from build123d import *

# Parameters (mm, degrees)
ESQUISSE1_W             = 90
ESQUISSE1_H             = 40
ESQUISSE1_R             = 5.05
ESQUISSE1_R_2           = 1.75
BOSS_EXTRU_1_DEPTH      = 10
ESQUISSE3_W             = 80
ESQUISSE3_H             = 40
ENL_V_MAT_EXTRU_3_DEPTH = 5
ESQUISSE4_R             = 1.75
BOSS_EXTRU_2_DEPTH      = 10
ESQUISSE2_R             = 1.75
ENL_V_MAT_EXTRU_1_DEPTH = 5
ENL_V_START             = -85
ESQUISSE2_2_R           = 1.75
ENL_V_MAT_EXTRU_2_DEPTH = 5
BOSS_EXTRU_3_START      = 10
ESQUISSE5_W             = 10
ESQUISSE5_H             = 50
ESQUISSE5_R             = 1.75
BOSS_EXTRU_3_DEPTH      = 10
BOSS_EXTRU_4_START      = -100
ESQUISSE5_2_W           = 10
ESQUISSE5_2_H           = 50
ESQUISSE5_2_R           = 1.75
BOSS_EXTRU_4_DEPTH      = 10
ESQUISSE6_R             = 1.75
ENL_V_MAT_EXTRU_4_DEPTH = 10
ESQUISSE7_R             = 5.05
ESQUISSE7_R_2           = 4.05
BOSS_EXTRU_5_DEPTH      = 2
ESQUISSE8_R             = 8
ESQUISSE8_R_2           = 5.05
BOSS_EXTRU_6_DEPTH      = 1.8


with BuildPart() as part:
    # Esquisse1 → Boss.-Extru.1 (new body)
    with BuildSketch(Plane.XY):
        with Locations((45, 20)):
            Rectangle(ESQUISSE1_W, ESQUISSE1_H)
        with Locations((45, 19)):
            Circle(ESQUISSE1_R, mode=Mode.SUBTRACT)
        with Locations((15, 35)):
            Circle(ESQUISSE1_R_2, mode=Mode.SUBTRACT)
        with Locations((25, 35)):
            Circle(ESQUISSE1_R_2, mode=Mode.SUBTRACT)
        with Locations((35, 35)):
            Circle(ESQUISSE1_R_2, mode=Mode.SUBTRACT)
        with Locations((55, 35)):
            Circle(ESQUISSE1_R_2, mode=Mode.SUBTRACT)
        with Locations((65, 35)):
            Circle(ESQUISSE1_R_2, mode=Mode.SUBTRACT)
        with Locations((75, 35)):
            Circle(ESQUISSE1_R_2, mode=Mode.SUBTRACT)
        with Locations((15, 25)):
            Circle(ESQUISSE1_R_2, mode=Mode.SUBTRACT)
        with Locations((25, 25)):
            Circle(ESQUISSE1_R_2, mode=Mode.SUBTRACT)
        with Locations((65, 25)):
            Circle(ESQUISSE1_R_2, mode=Mode.SUBTRACT)
        with Locations((75, 25)):
            Circle(ESQUISSE1_R_2, mode=Mode.SUBTRACT)
        with Locations((15, 15)):
            Circle(ESQUISSE1_R_2, mode=Mode.SUBTRACT)
        with Locations((25, 15)):
            Circle(ESQUISSE1_R_2, mode=Mode.SUBTRACT)
        with Locations((65, 15)):
            Circle(ESQUISSE1_R_2, mode=Mode.SUBTRACT)
        with Locations((75, 15)):
            Circle(ESQUISSE1_R_2, mode=Mode.SUBTRACT)
        with Locations((15, 5)):
            Circle(ESQUISSE1_R_2, mode=Mode.SUBTRACT)
        with Locations((25, 5)):
            Circle(ESQUISSE1_R_2, mode=Mode.SUBTRACT)
        with Locations((35, 5)):
            Circle(ESQUISSE1_R_2, mode=Mode.SUBTRACT)
        with Locations((45, 5)):
            Circle(ESQUISSE1_R_2, mode=Mode.SUBTRACT)
        with Locations((55, 5)):
            Circle(ESQUISSE1_R_2, mode=Mode.SUBTRACT)
        with Locations((65, 5)):
            Circle(ESQUISSE1_R_2, mode=Mode.SUBTRACT)
        with Locations((75, 5)):
            Circle(ESQUISSE1_R_2, mode=Mode.SUBTRACT)
    extrude(amount=BOSS_EXTRU_1_DEPTH)

    # Esquisse3 → Enlèv. mat.-Extru.3 (cut)
    with BuildSketch(Plane.XY.offset(10)):
        with Locations((45, 20)):
            Rectangle(ESQUISSE3_W, ESQUISSE3_H)
    extrude(amount=-ENL_V_MAT_EXTRU_3_DEPTH, mode=Mode.SUBTRACT)

    # Esquisse4 → Boss.-Extru.2 (add)
    with BuildSketch(Plane.XZ):
        Polygon((0, 0), (0, 10), (10, 10), (10, 5), (80, 5), (80, 10), (90, 10), (90, 0), align=None)
        with Locations((5, 5)):
            Circle(ESQUISSE4_R, mode=Mode.SUBTRACT)
        with Locations(Location((85, 5, 0), (0, 0, 180))):
            Circle(ESQUISSE4_R, mode=Mode.SUBTRACT)
    extrude(amount=BOSS_EXTRU_2_DEPTH)

    # Esquisse2 → Enlèv. mat.-Extru.1 (cut)
    with BuildSketch(Plane(origin=(90, 0, 0), x_dir=(0, 0, -1), z_dir=(1, 0, 0))):
        with Locations(Location((-5, 35, 0), (0, 0, 90))):
            Circle(ESQUISSE2_R)
        with Locations(Location((-5, 25, 0), (0, 0, 90))):
            Circle(ESQUISSE2_R)
        with Locations(Location((-5, 15, 0), (0, 0, 90))):
            Circle(ESQUISSE2_R)
        with Locations(Location((-5, 5, 0), (0, 0, 90))):
            Circle(ESQUISSE2_R)
        with Locations(Location((-5, -5, 0), (0, 0, 90))):
            Circle(ESQUISSE2_R)
    extrude(amount=-ENL_V_MAT_EXTRU_1_DEPTH, mode=Mode.SUBTRACT)

    # Esquisse2<2> → Enlèv. mat.-Extru.2 (cut)
    with BuildSketch(Plane(origin=(90, 0, 0), x_dir=(0, 0, -1), z_dir=(1, 0, 0)).offset(ENL_V_START)):
        with Locations(Location((-5, 35, 0), (0, 0, 90))):
            Circle(ESQUISSE2_2_R)
        with Locations(Location((-5, 25, 0), (0, 0, 90))):
            Circle(ESQUISSE2_2_R)
        with Locations(Location((-5, 15, 0), (0, 0, 90))):
            Circle(ESQUISSE2_2_R)
        with Locations(Location((-5, 5, 0), (0, 0, 90))):
            Circle(ESQUISSE2_2_R)
        with Locations(Location((-5, -5, 0), (0, 0, 90))):
            Circle(ESQUISSE2_2_R)
    extrude(amount=-ENL_V_MAT_EXTRU_2_DEPTH, mode=Mode.SUBTRACT)

    # Esquisse5 → Boss.-Extru.3 (add)
    with BuildSketch(Plane(origin=(90, 0, 0), x_dir=(0, 0, -1), z_dir=(1, 0, 0)).offset(BOSS_EXTRU_3_START)):
        with Locations((-5, 15)):
            Rectangle(ESQUISSE5_W, ESQUISSE5_H)
        with Locations(Location((-5, 35, 0), (0, 0, 90))):
            Circle(ESQUISSE5_R, mode=Mode.SUBTRACT)
        with Locations(Location((-5, 25, 0), (0, 0, 90))):
            Circle(ESQUISSE5_R, mode=Mode.SUBTRACT)
        with Locations(Location((-5, 15, 0), (0, 0, 90))):
            Circle(ESQUISSE5_R, mode=Mode.SUBTRACT)
        with Locations(Location((-5, 5, 0), (0, 0, 90))):
            Circle(ESQUISSE5_R, mode=Mode.SUBTRACT)
        with Locations(Location((-5, -5, 0), (0, 0, 90))):
            Circle(ESQUISSE5_R, mode=Mode.SUBTRACT)
    extrude(amount=-BOSS_EXTRU_3_DEPTH)

    # Esquisse5<2> → Boss.-Extru.4 (add)
    with BuildSketch(Plane(origin=(90, 0, 0), x_dir=(0, 0, -1), z_dir=(1, 0, 0)).offset(BOSS_EXTRU_4_START)):
        with Locations((-5, 15)):
            Rectangle(ESQUISSE5_2_W, ESQUISSE5_2_H)
        with Locations(Location((-5, 35, 0), (0, 0, 90))):
            Circle(ESQUISSE5_2_R, mode=Mode.SUBTRACT)
        with Locations(Location((-5, 25, 0), (0, 0, 90))):
            Circle(ESQUISSE5_2_R, mode=Mode.SUBTRACT)
        with Locations(Location((-5, 15, 0), (0, 0, 90))):
            Circle(ESQUISSE5_2_R, mode=Mode.SUBTRACT)
        with Locations(Location((-5, 5, 0), (0, 0, 90))):
            Circle(ESQUISSE5_2_R, mode=Mode.SUBTRACT)
        with Locations(Location((-5, -5, 0), (0, 0, 90))):
            Circle(ESQUISSE5_2_R, mode=Mode.SUBTRACT)
    extrude(amount=BOSS_EXTRU_4_DEPTH)

    # Esquisse6 → Enlèv. mat.-Extru.4 (cut)
    with BuildSketch(Plane(origin=(0, 0, 0), x_dir=(-1, 0, 0), z_dir=(0, 0, -1))):
        with Locations((-95, 35)):
            Circle(ESQUISSE6_R)
        with Locations((5, 35)):
            Circle(ESQUISSE6_R)
        with Locations((5, 25)):
            Circle(ESQUISSE6_R)
        with Locations((5, 15)):
            Circle(ESQUISSE6_R)
        with Locations((5, 5)):
            Circle(ESQUISSE6_R)
        with Locations((5, -5)):
            Circle(ESQUISSE6_R)
        with Locations((-95, 25)):
            Circle(ESQUISSE6_R)
        with Locations((-95, 15)):
            Circle(ESQUISSE6_R)
        with Locations((-95, 5)):
            Circle(ESQUISSE6_R)
        with Locations((-95, -5)):
            Circle(ESQUISSE6_R)
    extrude(amount=-ENL_V_MAT_EXTRU_4_DEPTH, mode=Mode.SUBTRACT)

    # Esquisse7 → Boss.-Extru.5 (add)
    with BuildSketch(Plane(origin=(0, 0, 0), x_dir=(-1, 0, 0), z_dir=(0, 0, -1))):
        with Locations(Location((-45, 19, 0), (0, 0, 180))):
            Circle(ESQUISSE7_R)
        with Locations((-45, 19)):
            Circle(ESQUISSE7_R_2, mode=Mode.SUBTRACT)
    extrude(amount=-BOSS_EXTRU_5_DEPTH)

    # Esquisse8 → Boss.-Extru.6 (add)
    with BuildSketch(Plane.XY.offset(5)):
        with Locations((45, 19)):
            Circle(ESQUISSE8_R)
        with Locations((45, 19)):
            Circle(ESQUISSE8_R_2, mode=Mode.SUBTRACT)
    extrude(amount=BOSS_EXTRU_6_DEPTH)


solid = part.part
Geometry check sheet. Reference: the model listing, model coordinates, mm. A direction names the side the tool comes from. Round coordinates to 2 decimals unless told otherwise and drop trailing zeros. Loops run counter-clockwise (first coordinate to the right, second up) from the corner with the lowest first, then second, coordinate; pieces in that order, holes last. Notation, with made-up numbers: (83.25, -28) -> (117.25, -28) arc R29 cw to (117.25, 6) -> close; hole circle Ø1 at (16, 87). An arc over 180 degrees is marked (long way). Answer as a JSON object with one key per item and string values. Group by question number.
Item 1: Depth check by flat-ended pin: pin 1 Ø13 at (x, y) = (45, 19) entering from +Z; pin 2 Ø3 at (y, z) = (35, 5) entering from -X; pin 3 Ø2 at (x, y) = (47, 22.5) entering from -Z; pin 4 Ø4 at (x, z) = (82.5, 8) entering from +Y. Enter the tip coordinate at first touch or a pass-through.
Item 2: Thickness scan on line 1 along Y through (x, z) = (15, 2.3); line 2 along X through (y, z) = (15, 7.75); line 3 along X through (y, z) = (-5, 3.1). Record the ranges inside material, lowest first.
Item 3: Release check for a two-part mould opening along Z. For faces 4 (the face through (44.2, 14.6, 0)), 5 (the face through (66.669, 25.526, 2.465)), 6 (the face through (41, 17, 2)), 7 (the face through (1.04, 3.25, 5.08)) record: pulls with the +Z half, pulls with the -Z half, needs draft (parallel to the pull), parting line crosses it, or undercut.
Item 4: Cross-section at A-A, the plane y = -2. Record the cut outline in (x, z).
Item 5: Cross-section at C-C, the plane x = 35. Record the cut outline in (y, z).
Item 6: Cross-section at B-B, the plane x = 75. Record the cut outline in (y, z), plus the area to 3 significant figures.
Item 7: Set-up check for faces 1 (the face through (96.75, 25.08, 1.91)), 2 (the face through (83.331, -4.93, 4.474)), 3 (the face through (85, 20, 8)): record each of +Z, -Z, +X, -X, +Y, -Y from which the full face is reachable in a straight line by a thin tool's end or side.
Item 8: Cross-section at D-D, the plane y = 5. Count the separate pieces of the cut face and the enclosed holes in it, plus the area to 3 significant figures.
Determined:
{
 "1": {"pin 1": "stops at z = 6.8", "pin 2": "stops at x = 5", "pin 3": "stops at z = 0", "pin 4": "stops at y = 0"},
 "2": {"line 1": "y = -10 to 3.25, 6.75 to 13.25, 16.75 to 23.25, 26.75 to 33.25, 36.75 to 40", "line 2": "x = -10 to -6.75, -3.25 to 5, 85 to 93.25, 96.75 to 100", "line 3": "x = -10 to -6.75, -3.25 to 93.25, 96.75 to 100"},
 "3": {"face 4": "pulls with the -Z half", "face 5": "needs draft", "face 6": "pulls with the +Z half", "face 7": "undercut"},
 "4": {"outline": "(-10, 0) -> (100, 0) -> (100, 10) -> (80, 10) -> (80, 5) -> (10, 5) -> (10, 10) -> (-10, 10) -> close; hole circle Ø3.5 at (5, 5); hole circle Ø3.5 at (85, 5)"},
 "5": {"outline": "(-10, 0) -> (3.25, 0) -> (3.25, 5) -> (-10, 5) -> close; (6.75, 0) -> (33.25, 0) -> (33.25, 5) -> (6.75, 5) -> close; (36.75, 0) -> (40, 0) -> (40, 5) -> (36.75, 5) -> close"},
 "6": {"outline": "(-10, 0) -> (3.25, 0) -> (3.25, 5) -> (-10, 5) -> close; (6.75, 0) -> (13.25, 0) -> (13.25, 5) -> (6.75, 5) -> close; (16.75, 0) -> (23.25, 0) -> (23.25, 5) -> (16.75, 5) -> close; (26.75, 0) -> (33.25, 0) -> (33.25, 5) -> (26.75, 5) -> close; (36.75, 0) -> (40, 0) -> (40, 5) -> (36.75, 5) -> close", "area": "180 mm²"},
 "7": {"face 1": "+Z, -Z", "face 2": "-Y", "face 3": "+Z, +Y"},
 "8": {"separate pieces": "14", "enclosed holes": "0", "area": "427 mm²"}
}
